from build123d import *

# Parameters (mm, degrees)
SKETCH1_W           = 18.67
SKETCH1_H           = 20.27
BOSS_EXTRUDE1_DEPTH = 10
SKETCH2_W           = 18.67
SKETCH2_H           = 20.27
SKETCH2_W_2         = 16.47
SKETCH2_H_2         = 18.07
CUT_EXTRUDE1_DEPTH  = 5
SKETCH7_W           = 18.67
SKETCH7_H           = 20.27
SKETCH7_W_2         = 14.47
SKETCH7_H_2         = 16.07
CUT_EXTRUDE5_DEPTH  = 5
SKETCH3_W           = 10.47
SKETCH3_H           = 12.07
CUT_EXTRUDE2_DEPTH  = 16
CUT_EXTRUDE3_START  = -10
SKETCH4_W           = 2
SKETCH4_H           = 13.07
CUT_EXTRUDE3_DEPTH  = 10
SKETCH6_W           = 3.5
SKETCH6_H           = 12.07
BOSS_EXTRUDE2_DEPTH = 5
SKETCH5_W           = 0.5
SKETCH5_H           = 1
CUT_EXTRUDE4_DEPTH  = 7


with BuildPart() as part:
    # Sketch1 → Boss-Extrude1 (new body, symmetric)
    with BuildSketch(Plane(origin=(0, 0, 0), x_dir=(1, 0, 0), z_dir=(0, 1, 0))):
        Rectangle(SKETCH1_W, SKETCH1_H)
    extrude(amount=BOSS_EXTRUDE1_DEPTH, both=True)

    # Sketch2 → Cut-Extrude1 (cut)
    with BuildSketch(Plane(origin=(0, 10, 0), x_dir=(1, 0, 0), z_dir=(0, 1, 0))):
        Rectangle(SKETCH2_W, SKETCH2_H)
        Rectangle(SKETCH2_W_2, SKETCH2_H_2, mode=Mode.SUBTRACT)
    extrude(amount=-CUT_EXTRUDE1_DEPTH, mode=Mode.SUBTRACT)

    # Sketch7 → Cut-Extrude5 (cut)
    with BuildSketch(Plane.XZ.offset(10)):
        Rectangle(SKETCH7_W, SKETCH7_H)
        Rectangle(SKETCH7_W_2, SKETCH7_H_2, mode=Mode.SUBTRACT)
    extrude(amount=-CUT_EXTRUDE5_DEPTH, mode=Mode.SUBTRACT)

    # Sketch3 → Cut-Extrude2 (cut)
    with BuildSketch(Plane.XZ.offset(10)):
        Rectangle(SKETCH3_W, SKETCH3_H)
    extrude(amount=-CUT_EXTRUDE2_DEPTH, mode=Mode.SUBTRACT)

    # Sketch4 → Cut-Extrude3 (cut)
    with BuildSketch(Plane(origin=(0, 10, 0), x_dir=(1, 0, 0), z_dir=(0, 1, 0)).offset(CUT_EXTRUDE3_START)):
        with Locations((-4.735, 0)):
            Rectangle(SKETCH4_W, SKETCH4_H)
        with Locations((4.735, 0)):
            Rectangle(SKETCH4_W, SKETCH4_H)
    extrude(amount=CUT_EXTRUDE3_DEPTH, mode=Mode.SUBTRACT)

    # Sketch6 → Boss-Extrude2 (add)
    with BuildSketch(Plane.XZ.offset(-6)):
        Rectangle(SKETCH6_W, SKETCH6_H)
    extrude(amount=BOSS_EXTRUDE2_DEPTH)

    # Sketch5 → Cut-Extrude4 (cut)
    with BuildSketch(Plane(origin=(0, 10, 0), x_dir=(1, 0, 0), z_dir=(0, 1, 0))):
        with Locations((0, -6.1)):
            Rectangle(SKETCH5_W, SKETCH5_H)
        with Locations((0, 6.1)):
            Rectangle(SKETCH5_W, SKETCH5_H)
    extrude(amount=-CUT_EXTRUDE4_DEPTH, mode=Mode.SUBTRACT)


solid = part.part
The listing builds one solid part. Answer for the finished solid, in the listing's coordinates (mm). A direction names the side the tool comes from. Coordinates: 2 decimals unless noted, no trailing zeros. Loops run counter-clockwise (first coordinate to the right, second up) from the corner with the lowest first, then second, coordinate; pieces in that order, holes last. Notation, with made-up numbers: (75.5, 46.25) -> (103.5, 46.25) arc R11 cw to (103.5, 57.25) -> close; hole circle Ø10 at (75, 80.5). An arc over 180 degrees is marked (long way). Answer in a Markdown table with one row per item. Add a question column.
1. The part is cut by section D-D, the plane y = -5.5. Write down the section's boundary in (x, z) (3 decimals).
2. For faces 4 (the flat face through (0, -8, 8.035)), 5 (the flat face through (0, 8, 9.035)), 6 (the flat face through (5.4, 0, 0)), 7 (the flat face through (7.235, -8, 0)), 8 (the flat face through (-7.235, -8, 0)), determine the directions among +Z, -Z, +X, -X, +Y, -Y from which every point of the face is accessible in a straight line to the end or side of a thin tool.
3. Determine the mould class of faces 1 (the flat face through (9.335, 0, 0)), 2 (the flat face through (0.25, 7, -6)), 3 (the flat face through (0, 0, -10.135)) for opening direction X: +X half, -X half, draft (parallel to the pull), parting line (faces both ways), or undercut.
4. Flat-ended cylindrical pins translate along their axes: P1, Ø5, axis at x = -1, z = 5, coming from the -Y side; P2, Ø4, axis at y = -8.5, z = -3, coming from the -X side (3 decimals); P3, Ø1.5, axis at y = 8, z = 3.5, coming from the -X side (3 decimals); P4, Ø0.6, axis at x = 3, z = -0.5, coming from the -Y side. Find the tip coordinate at first contact, or state that the pin passes through.
5. Consider line 1 (X direction, y = 4.5, z = -2.5) (3 decimals); line 2 (X direction, y = 7.25, z = -4.25) (3 decimals); line 3 (Z direction, x = -4.75, y = -2.25) (3 decimals). Determine where each line is inside the solid, lowest interval first. Write a range as [from, to].
6. The part is cut by section B-B, the plane y = 4.5. Write down the section's boundary in (x, z) (3 decimals), then the cut area to 3 significant figures.
7. The part is cut by section A-A, the plane z = -4. Write down the section's boundary in (x, y) (3 decimals).
8. The part is cut by section C-C, the plane x = -4.75. Write down the section's boundary in (y, z) (3 decimals), then the cut area to 3 significant figures.
Answer below:
| question | item | result |
|---|---|---|
| 1 | outline | (-7.235, -8.035) -> (7.235, -8.035) -> (7.235, 8.035) -> (-7.235, 8.035) -> close; hole (-5.235, -6.035) -> (5.235, -6.035) -> (5.235, 6.035) -> (-5.235, 6.035) -> close |
| 2 | face 4 | +Z, +X, -X, -Y |
| 2 | face 5 | +Z, +X, -X, +Y |
| 2 | face 6 | +Y |
| 2 | face 7 | +Z, -Z, +X, -Y |
| 2 | face 8 | +Z, -Z, -X, -Y |
| 3 | face 1 | +X half |
| 3 | face 2 | undercut |
| 3 | face 3 | draft |
| 4 | P1 | y = -10 |
| 4 | P2 | x = -7.235 |
| 4 | P3 | x = -8.235 |
| 4 | P4 | y = 6 |
| 5 | line 1 | [-9.335, -5.735], [-1.75, 1.75], [5.735, 9.335] |
| 5 | line 2 | [-8.235, -5.735], [-3.735, 3.735], [5.735, 8.235] |
| 5 | line 3 | [-10.135, -6.035], [6.035, 10.135] |
| 6 | outline | (-9.335, -10.135) -> (9.335, -10.135) -> (9.335, 10.135) -> (-9.335, 10.135) -> close; hole (-5.735, -6.535) -> (-3.735, -6.535) -> (-3.735, -6.035) -> (-1.75, -6.035) -> (-1.75, 6.035) -> (-3.735, 6.035) -> (-3.735, 6.535) -> (-5.735, 6.535) -> close; hole (-0.25, -6.6) -> (0.25, -6.6) -> (0.25, -5.6) -> (-0.25, -5.6) -> close; hole (-0.25, 5.6) -> (0.25, 5.6) -> (0.25, 6.6) -> (-0.25, 6.6) -> close; hole (1.75, -6.035) -> (3.735, -6.035) -> (3.735, -6.535) -> (5.735, -6.535) -> (5.735, 6.535) -> (3.735, 6.535) -> (3.735, 6.035) -> (1.75, 6.035) -> close |
| 6 | area | 277 mm2 |
| 7 | outline | (-9.335, -5) -> (-7.235, -5) -> (-7.235, -10) -> (-5.235, -10) -> (-5.235, 0) -> (-5.735, 0) -> (-5.735, 10) -> (-8.235, 10) -> (-8.235, 5) -> (-9.335, 5) -> close; (-3.735, 6) -> (-1.75, 6) -> (-1.75, 1) -> (1.75, 1) -> (1.75, 6) -> (3.735, 6) -> (3.735, 10) -> (-3.735, 10) -> close; (5.235, -10) -> (7.235, -10) -> (7.235, -5) -> (9.335, -5) -> (9.335, 5) -> (8.235, 5) -> (8.235, 10) -> (5.735, 10) -> (5.735, 0) -> (5.235, 0) -> close |
| 8 | outline | (-10, -8.035) -> (-5, -8.035) -> (-5, -10.135) -> (5, -10.135) -> (5, -9.035) -> (10, -9.035) -> (10, -6.535) -> (0, -6.535) -> (0, -6.035) -> (-10, -6.035) -> close; (-10, 6.035) -> (0, 6.035) -> (0, 6.535) -> (10, 6.535) -> (10, 9.035) -> (5, 9.035) -> (5, 10.135) -> (-5, 10.135) -> (-5, 8.035) -> (-10, 8.035) -> close |
| 8 | area | 122 mm2 |
